```python
from build123d import *

# Parameters (mm, degrees)
SKETCH2_R                = 40
BOSS_EXTRUDE1_DEPTH      = 10
EXTRUDE_THIN1_DEPTH      = 20
EXTRUDE_THIN1_DEPTH_BACK = 10
SKETCH3_R                = 50
SKETCH3_R_2              = 40
SKETCH4_OUTSIDE_W        = 130.914
SKETCH4_OUTSIDE_H        = 130.914
CUT_EXTRUDE1_DEPTH       = 77.811457479
SKETCH5_R                = 3
CUT_EXTRUDE2_DEPTH       = 75.893257373


with BuildPart() as part:
    # Sketch2 → Boss-Extrude1 (new body)
    with BuildSketch(Plane(origin=(0, 0, 0), x_dir=(1, 0, 0), z_dir=(0, 1, 0))):
        with Locations(Location((0, 0, 0), (0, 0, 270))):
            Circle(SKETCH2_R)
    extrude(amount=BOSS_EXTRUDE1_DEPTH)

    # Sketch3 → Extrude-Thin1 (add, two sides: drawn at the far end of the back side and taken through both)
    with BuildSketch(Plane.XZ.offset(-EXTRUDE_THIN1_DEPTH_BACK)):
        Circle(SKETCH3_R)
        Circle(SKETCH3_R_2, mode=Mode.SUBTRACT)
    extrude(amount=EXTRUDE_THIN1_DEPTH + EXTRUDE_THIN1_DEPTH_BACK)

    # Sketch4 outside → Cut-Extrude1 (cut, through all)
    with BuildSketch(Plane(origin=(0, 10, 0), x_dir=(1, 0, 0), z_dir=(0, 1, 0))):
        Rectangle(SKETCH4_OUTSIDE_W, SKETCH4_OUTSIDE_H)
        Polygon((54.270925304, 0), (27.135462652, 47), (-27.135462652, 47), (-54.270925304, 0), (-27.135462652, -47), (27.135462652, -47), align=None, mode=Mode.SUBTRACT)
    extrude(amount=-CUT_EXTRUDE1_DEPTH, mode=Mode.SUBTRACT)

    # Sketch5 → Cut-Extrude2 (cut, through all)
    with BuildSketch(Plane(origin=(0, 10, 0), x_dir=(1, 0, 0), z_dir=(0, 1, 0))):
        with Locations(Location((0, 25, 0), (0, 0, 270))):
            Circle(SKETCH5_R)
        with Locations(Location((21.650635095, 12.5, 0), (0, 0, 270))):
            Circle(SKETCH5_R)
        with Locations(Location((21.650635095, -12.5, 0), (0, 0, 270))):
            Circle(SKETCH5_R)
        with Locations(Location((0, -25, 0), (0, 0, 270))):
            Circle(SKETCH5_R)
        with Locations(Location((-21.650635095, -12.5, 0), (0, 0, 270))):
            Circle(SKETCH5_R)
        with Locations(Location((-21.650635095, 12.5, 0), (0, 0, 270))):
            Circle(SKETCH5_R)
    extrude(amount=-CUT_EXTRUDE2_DEPTH, mode=Mode.SUBTRACT)


solid = part.part
```
For this review, take the finished solid that the model builds, in its own axes (mm). A direction names the side the tool comes from. Give positions to 0.01 mm unless a question says otherwise; leave off trailing zeros. Loops run counter-clockwise (first coordinate to the right, second up) from the corner with the lowest first, then second, coordinate; pieces in that order, holes last. Notation, with made-up numbers: M 69,-17.5 L 77,-17.5 A28 cw 77,1.5 Z; hole C 32,62 d8. An arc over 180 degrees is marked long. One line per item, written item: value. Start each with the question number.
Q1. For L1, parallel to Z at x = 0, y = -6.75; L2, parallel to Y at x = -8, z = -26; L3, parallel to X at y = -10.5, z = 21, list the stretches that pass through material, from the lowest coordinate up.
Q2. Clearance check with flat-ended pins moving along their axes: pin 1 Ø6 at (y, z) = (-10.5, -11.5) entering from +X; pin 2 Ø1 at (x, y) = (20.5, -16.5) entering from -Z; pin 3 Ø5.5 at (x, z) = (21.65, 12.5) entering from +Y; pin 4 Ø12 at (x, y) = (-37, -1) entering from -Z. State where each tip first meets the part, or that it passes through.
Q3. Add section C-C (z = 0). Give the boundary of the cut face in (x, y), and give its area (3 significant figures).
Q4. Add section B-B (z = 25). Give the boundary of the cut face in (x, y), and give its area (3 significant figures).
Q5. Machinability: for faces 1 (the face through (11, -20, 39)), 2 (the face through (36.95, -9.86, -15.32)), which of the approach directions +Z, -Z, +X, -X, +Y, -Y give a long, thin tool a straight path to every point of the face, cutting with its end or side? Answer none if there is none.
Q6. Draft analysis for pull direction Z (two halves, no side actions). For faces 3 (the face through (-24.58, 5.07, 11.85)), 4 (the face through (0, -5, 47)), 5 (the face through (-50, -5, 0)), state which applies: released by +Z, released by -Z, zero draft, split by the parting line, or undercut.
Q7. Add section A-A (y = -12.5). Give the boundary of the cut face in (x, z), and give its area (3 significant figures).
Q8. Add section D-D (y = 6). Give the boundary of the cut face in (x, z), and give its area (3 significant figures).
Reply:
1. L1: -47 to -40, 40 to 47
1. L2: 0 to 10
1. L3: -42.15 to -34.04, 34.04 to 42.15
2. pin 1: x = 49.27
2. pin 2: z = -45.83
2. pin 3: through
2. pin 4: z = -39.23
3. outline: M -50,-20 L -40,-20 L -40,0 L 40,0 L 40,-20 L 50,-20 L 50,10 L -50,10 Z
3. area: 1,400 mm²
4. outline: M -39.84,-20 L -31.22,-20 L -31.22,0 L -3,0 L -3,10 L -39.84,10 Z; M 3,0 L 31.22,0 L 31.22,-20 L 39.84,-20 L 39.84,10 L 3,10 Z
4. area: 1,080 mm²
5. face 1: +Z, -Z, +X, -X, -Y
5. face 2: -Y
6. face 3: undercut
6. face 4: released by +Z
6. face 5: split by the parting line
7. outline: M -49.23,-8.73 L -32.17,-38.27 A50 ccw -17.06,-47 L 17.06,-47 A50 ccw 32.17,-38.27 L 49.23,-8.73 A50 ccw 49.23,8.73 L 32.17,38.27 A50 ccw 17.06,47 L -17.06,47 A50 ccw -32.17,38.27 L -49.23,8.73 A50 ccw Z; hole C 0,0 d80
7. area: 2,420 mm²
8. outline: M -49.23,-8.73 L -32.17,-38.27 A50 ccw -17.06,-47 L 17.06,-47 A50 ccw 32.17,-38.27 L 49.23,-8.73 A50 ccw 49.23,8.73 L 32.17,38.27 A50 ccw 17.06,47 L -17.06,47 A50 ccw -32.17,38.27 L -49.23,8.73 A50 ccw Z; hole C -21.65,-12.5 d6; hole C -21.65,12.5 d6; hole C 0,-25 d6; hole C 0,25 d6; hole C 21.65,-12.5 d6; hole C 21.65,12.5 d6
8. area: 7,270 mm²
